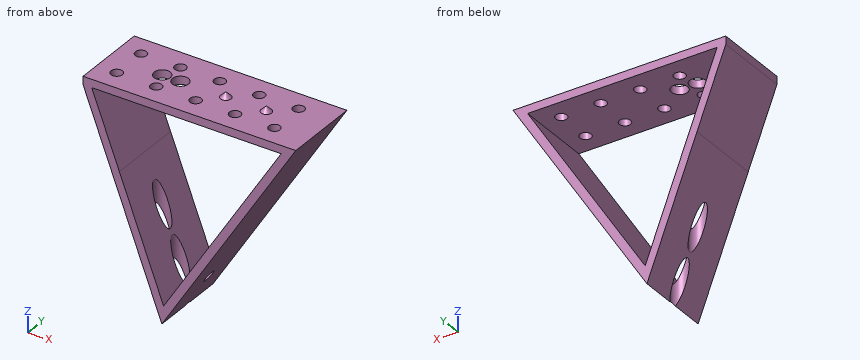
```python
from build123d import *

# Parameters (mm, degrees)
SKETCH1_W           = 49
SKETCH1_H           = 19
BOSS_EXTRUDE1_DEPTH = 2
SKETCH3_R           = 1.4
CUT_EXTRUDE1_DEPTH  = 27.353367906
SKETCH5_R           = 2
CUT_EXTRUDE2_DEPTH  = 10
SKETCH2_R           = 1.3
BOSS_EXTRUDE2_DEPTH = 2.5
BOSS_EXTRUDE3_DEPTH = 19
BOSS_EXTRUDE4_DEPTH = 19
SKETCH7_R           = 2
CUT_EXTRUDE3_DEPTH  = 60.183519481
SKETCH8_R           = 1.5
CUT_EXTRUDE4_DEPTH  = 2


# Read off the part's stored shape, not the designer's step: Draft1
with BuildPart() as part:
    # Sketch1 → Boss-Extrude1 (new body)
    with BuildSketch(Plane.XY):
        Rectangle(SKETCH1_W, SKETCH1_H)
    extrude(amount=BOSS_EXTRUDE1_DEPTH)

    # Sketch3 → Cut-Extrude1 (cut, through all)
    with BuildSketch(Plane.XY.offset(2)):
        with Locations((19.5, 4.5)):
            Circle(SKETCH3_R)
        with Locations((9.75, 4.5)):
            Circle(SKETCH3_R)
        with Locations((0, 4.5)):
            Circle(SKETCH3_R)
        with Locations((-9.75, 4.5)):
            Circle(SKETCH3_R)
        with Locations((-19.5, 4.5)):
            Circle(SKETCH3_R)
        with Locations((-19.5, -4.5)):
            Circle(SKETCH3_R)
        with Locations((-9.75, -4.5)):
            Circle(SKETCH3_R)
        with Locations((0, -4.5)):
            Circle(SKETCH3_R)
        with Locations((9.75, -4.5)):
            Circle(SKETCH3_R)
        with Locations((19.5, -4.5)):
            Circle(SKETCH3_R)
    extrude(amount=-CUT_EXTRUDE1_DEPTH, mode=Mode.SUBTRACT)

    # Sketch5 → Cut-Extrude2 (cut)
    with BuildSketch(Plane.XY.offset(2)):
        with Locations((-6.75, 0)):
            Circle(SKETCH5_R)
        with Locations((-11.25, 0)):
            Circle(SKETCH5_R)
    extrude(amount=-CUT_EXTRUDE2_DEPTH, mode=Mode.SUBTRACT)

    # Sketch2 → Boss-Extrude2 (add)
    with BuildSketch(Plane.XY.offset(2)):
        with Locations((4.5, 0)):
            Circle(SKETCH2_R)
        with Locations((14.5, 0)):
            Circle(SKETCH2_R)
    extrude(amount=BOSS_EXTRUDE2_DEPTH)

    # Draft1 outline → Draft1 (revolve, cut)
    with BuildSketch(Plane(origin=(4.5, 0, 0), x_dir=(1, 0, 0), z_dir=(0, -1, 0))):
        Polygon((1.3, 2), (1.3, 4.5), (0, 4.5), (0, 3.3), align=None)
    revolve(axis=Axis((4.5, 0, 0), (0, 0, 1)), mode=Mode.SUBTRACT)

    # Draft1 2 outline → Draft1 2 (revolve, cut)
    with BuildSketch(Plane(origin=(14.5, 0, 0), x_dir=(1, 0, 0), z_dir=(0, -1, 0))):
        Polygon((1.3, 2), (1.3, 4.5), (0, 4.5), (0, 3.3), align=None)
    revolve(axis=Axis((14.5, 0, 0), (0, 0, 1)), mode=Mode.SUBTRACT)

    # Sketch4 → Boss-Extrude3 (add)
    with BuildSketch(Plane.XZ.offset(9.5)):
        Polygon((-24.5, 0), (-17.386542933, -18.692210371), (-15.517321896, -17.980864664), (-22.360071163, 0), align=None)
    extrude(amount=-BOSS_EXTRUDE3_DEPTH)

    # Sketch6 → Boss-Extrude4 (add)
    with BuildSketch(Plane.XZ.offset(9.5)):
        Polygon((-15.517321896, -17.980864664), (-4.576428495, -46.730525927), (24.5, 0), (24.5, 2), (28.099977552, 2), (-5.010300383, -51.213574761), (-17.386542933, -18.692210371), align=None)
    extrude(amount=-BOSS_EXTRUDE4_DEPTH)

    # Sketch7 → Cut-Extrude3 (cut, through all)
    with BuildSketch(Plane(origin=(0, 0, 0), x_dir=(-1, 0, 0), z_dir=(0, 0, -1))):
        with Locations(Location((11.25, 0, 0), (0, 0, 180))):
            Circle(SKETCH7_R)
        with Locations(Location((6.75, 0, 0), (0, 0, 180))):
            Circle(SKETCH7_R)
    extrude(amount=CUT_EXTRUDE3_DEPTH, mode=Mode.SUBTRACT)

    # Sketch8 → Cut-Extrude4 (cut)
    with BuildSketch(Plane(origin=(19.36021452, 0, -12.046213518), x_dir=(-0.5282973915815173, 0, -0.849059400777216), z_dir=(0.8490594007772159, 0, -0.5282973915815172))):
        with Locations((36.130295721, 0)):
            Circle(SKETCH8_R)
    extrude(amount=-CUT_EXTRUDE4_DEPTH, mode=Mode.SUBTRACT)


solid = part.part
```
For this review, take the finished solid that the model builds, in its own axes (mm). Coordinates: 2 decimals unless noted, no trailing zeros. Write each loop counter-clockwise with the first axis right and the second up, starting at its lowest first coordinate (ties: lowest second). Pieces come first, ordered by that corner, then holes. Notation, with made-up numbers: (-32, 55) - (18, 55) arc R36 ccw to (18, 94) - close; hole circle Ø4 at (-16, 1.5). An arc over 180 degrees is marked (long way). Put each result on its own line as item: value.
1. For pin 1 (3.5 mm diameter, centred on x = -19.5, y = 4.5, fed in from +Z); pin 2 (9.5 mm diameter, centred on x = 3, y = -4.5, fed in from -Z); pin 3 (3 mm diameter, centred on x = 9.75, y = 4.5, fed in from -Z), all flat-tipped, find the tip position at first contact; note any pin that passes through.
Values found:
pin 1: z = 2
pin 2: z = -45.97
pin 3: z = -29.9
2. Add section D-D, the plane x = 16.5. Give the boundary of the cut face in (y, z), then the cut area to 3 significant figures.
Values found:
outline: (-9.5, -16.64) - (9.5, -16.64) - (9.5, -12.86) - (-9.5, -12.86) - close; (-9.5, 0) - (9.5, 0) - (9.5, 2) - (-9.5, 2) - close
area: 110 mm²
3. Wall thickness on probe 1 along Y at (x, z) = (-19.5, 0.6); probe 2 along Z at (x, y) = (7, 6.25); probe 3 along X at (y, z) = (6.5, -38.5): over which ranges is each line inside the solid? List them lowest first.
Values found:
probe 1: -9.5 to -5.9, -3.1 to 3.1, 5.9 to 9.5
probe 2: -31.91 to -28.13, 0 to 2
probe 3: -9.85 to -7.71, 0.54 to 2.9
4. Add section C-C, the plane z = -16.5. Give the boundary of the cut face in (x, y), then the cut area to 3 significant figures.
Values found:
outline: (-18.22, -9.5) - (-16.08, -9.5) - (-16.08, 9.5) - (-18.22, 9.5) - close; (14.23, -9.5) - (16.59, -9.5) - (16.59, 9.5) - (14.23, 9.5) - close
area: 85.4 mm²
5. Add section A-A, the plane y = 8. Give the boundary of the cut face in (x, z).
Values found:
outline: (-24.5, 0) - (-5.01, -51.21) - (28.1, 2) - (-24.5, 2) - close; hole (-22.36, 0) - (-4.58, -46.73) - (24.5, 0) - close
6. Add section B-B, the plane x = 9.75. Give the boundary of the cut face in (y, z), then the cut area to 3 significant figures.
Values found:
outline: (-9.5, -27.49) - (9.5, -27.49) - (9.5, -23.71) - (-9.5, -23.71) - close; (-9.5, 0) - (-5.9, 0) - (-5.9, 2) - (-9.5, 2) - close; (-3.1, 0) - (3.1, 0) - (3.1, 2) - (-3.1, 2) - close; (5.9, 0) - (9.5, 0) - (9.5, 2) - (5.9, 2) - close
area: 98.7 mm²
